from build123d import *

# Parameters (mm, degrees)
BOSS_EXTRUDE1_DEPTH = 0.508
SKETCH2_R           = 2.695
SKETCH2_R_2         = 1.5
BOSS_EXTRUDE2_DEPTH = 5


with BuildPart() as part:
    # Sketch1 → Boss-Extrude1 (new body)
    with BuildSketch(Plane(origin=(0, 0, 0), x_dir=(1, 0, 0), z_dir=(0, 1, 0))):
        Polygon((1.847520861, -3.2), (3.695041723, 0), (1.847520861, 3.2), (-1.847520861, 3.2), (-3.695041723, 0), (-1.847520861, -3.2), align=None)
    extrude(amount=BOSS_EXTRUDE1_DEPTH)

    # Sketch2 → Boss-Extrude2 (add)
    with BuildSketch(Plane.XZ):
        Circle(SKETCH2_R)
        Circle(SKETCH2_R_2, mode=Mode.SUBTRACT)
    extrude(amount=-BOSS_EXTRUDE2_DEPTH)


solid = part.part
Geometry check sheet. Reference: the model listing, model coordinates, mm. A direction names the side the tool comes from. Round coordinates to 2 decimals unless told otherwise and drop trailing zeros. Write each loop counter-clockwise with the first axis right and the second up, starting at its lowest first coordinate (ties: lowest second). Pieces come first, ordered by that corner, then holes. Notation, with made-up numbers: (-16, 72.25) - (-7, 72.25) arc R10 ccw to (-7, 83.25) - close; hole circle Ø5 at (84.5, -11). An arc over 180 degrees is marked (long way). One line per item, written item: value.
1. Cross-section at C-C on y = 2.8. Record the boundary of the cut face in (x, z) (3 decimals), and give its area (3 significant figures).
The answers:
outline: circle Ø5.39 at (0, 0); hole circle Ø3 at (0, 0)
area: 15.7 mm^2
2. Cross-section at B-B on z = 2.5. Record the boundary of the cut face in (x, y).
The answers:
outline: (-2.25, 0) - (2.25, 0) - (2.25, 0.51) - (1.01, 0.51) - (1.01, 5) - (-1.01, 5) - (-1.01, 0.51) - (-2.25, 0.51) - close
3. Cross-section at D-D on z = 0.75. Record the boundary of the cut face in (x, y), and give its area (3 significant figures).
The answers:
outline: (-3.26, 0) - (3.26, 0) - (3.26, 0.51) - (2.59, 0.51) - (2.59, 5) - (1.3, 5) - (1.3, 0.51) - (-1.3, 0.51) - (-1.3, 5) - (-2.59, 5) - (-2.59, 0.51) - (-3.26, 0.51) - close
area: 14.9 mm^2
4. Depth check by flat-ended pin: pin 1 Ø1.5 at (y, z) = (3.5, 0.5) entering from +X (3 decimals). Enter the tip coordinate at first touch or a pass-through.
The answers:
pin 1: stops at x = 2.695
5. Mould release check, pull along X, two halves, no side actions. Record for faces 1 (the face through (-1.5, 2.72, 0.07)), 2 (the face through (-2.784, 0.25, 1.578)), 3 (the face through (0, 0, 0)): released by +X, released by -X, zero draft, split by the parting line, or undercut.
The answers:
face 1: undercut
face 2: released by -X
face 3: zero draft
6. Cross-section at A-A on x = 0. Record the boundary of the cut face in (y, z) (3 decimals), and give its area (3 significant figures).
The answers:
outline: (0, -3.2) - (0.508, -3.2) - (0.508, -2.695) - (5, -2.695) - (5, -1.5) - (0.508, -1.5) - (0.508, 1.5) - (5, 1.5) - (5, 2.695) - (0.508, 2.695) - (0.508, 3.2) - (0, 3.2) - close
area: 14.0 mm^2
7. Scan lines: L1, parallel to Z at x = 0, y = 1.6 (3 decimals); L2, parallel to Y at x = 2.25, z = -1.75; L3, parallel to X at y = 2.9, z = -1. Record each from-to range of solid material in increasing order.
The answers:
L1: z = -2.695 to -1.5, 1.5 to 2.695
L2: y = 0 to 0.51
L3: x = -2.5 to -1.12, 1.12 to 2.5
8. Set-up check for faces 4 (the face through (0, 0.508, 0)), 5 (the face through (-2.76, 0.25, -1.62)): record each of +Z, -Z, +X, -X, +Y, -Y from which the full face is reachable in a straight line by a thin tool's end or side.
The answers:
face 4: +Y
face 5: -Z, -X, +Y, -Y
